Read the model definition and answer for the solid it produces. Units are mm, in the model's axes. A direction names the side the tool comes from. Round coordinates to 2 decimals unless told otherwise and drop trailing zeros. Order: outer loops, then holes, each group sorted by start corner. A loop starts at its lowest first (then second) coordinate and runs counter-clockwise, first axis right, second up. Notation, with made-up numbers: (24.5, -29) -> (41.5, -29) arc R31 ccw to (41.5, 1) -> close; hole circle Ø10 at (50.5, 46.5). An arc over 180 degrees is marked (long way). Answer as a JSON object with one key per item and string values. Group by question number.
Item 1: The mould has two halves that part along Z. Classify faces 1 (the flat face through (16, -8, 48)), 2 (the flat face through (16, -8, 32)), 3 (the flat face through (32, -8, 24)), 4 (the flat face through (16, -8, 0)): pulls with the +Z half, pulls with the -Z half, needs draft (parallel to the pull), parting line crosses it, or undercut.
Item 2: Given P1, Ø4, axis at x = 20.5, z = 41.5, coming from the -Y side, flat-ended and moving along its own axis, determine where the tip first touches the part or whether it passes through.
Item 3: Section B-B, the plane z = 16 is taken. Write down the section's boundary in (x, y), plus the area to 3 significant figures.
Item 4: Section C-C, the plane x = 25 is taken. Write down the section's boundary in (y, z).
Item 5: Consider probe 1 along Z at (x, y) = (4.5, -11.5); probe 2 along X at (y, z) = (-11, 23.5); probe 3 along Y at (x, z) = (9, 39.5). Determine where each line is inside the solid, lowest interval first. Write a range as from..to.
Item 6: For faces 5 (the flat face through (0, -8, 24)), 6 (the flat face through (1, -8, 25)), determine the directions among +Z, -Z, +X, -X, +Y, -Y from which every point of the face is accessible in a straight line to the end or side of a thin tool.
Item 7: Section A-A, the plane y = -10.25 is taken. Write down the section's boundary in (x, z).
from build123d import *

# Parameters (mm, degrees)
F0_W     = 32
F0_H     = 48
F0_W_2   = 30
F0_H_2   = 15
F0_H_3   = 14
F1_DEPTH = 17
F2_W     = 32
F2_H     = 48
F3_DEPTH = 1


with BuildPart() as f1:
    # F0 (on Front) → F1 (new body)
    with BuildSketch(Plane.XZ):
        with Locations((16, 24)):
            Rectangle(F0_W, F0_H)
        with Locations((16, 9.5)):
            Rectangle(F0_W_2, F0_H_2, mode=Mode.SUBTRACT)
        with Locations((16, 25)):
            Rectangle(F0_W_2, F0_H_3, mode=Mode.SUBTRACT)
        with Locations((16, 40)):
            Rectangle(F0_W_2, F0_H_3, mode=Mode.SUBTRACT)
    extrude(amount=F1_DEPTH)

    # F2 (on Front) → F3 (join)
    with BuildSketch(Plane.XZ):
        with Locations((16, 24)):
            Rectangle(F2_W, F2_H)
    extrude(amount=-F3_DEPTH)


solid = f1.part
Values found:
{
 "1": {"face 1": "pulls with the +Z half", "face 2": "undercut", "face 3": "needs draft", "face 4": "pulls with the -Z half"},
 "2": {"P1": "y = 0"},
 "3": {"outline": "(0, -17) -> (1, -17) -> (1, 0) -> (31, 0) -> (31, -17) -> (32, -17) -> (32, 1) -> (0, 1) -> close", "area": "66.0 mm2"},
 "4": {"outline": "(-17, 0) -> (1, 0) -> (1, 48) -> (-17, 48) -> (-17, 47) -> (0, 47) -> (0, 33) -> (-17, 33) -> (-17, 32) -> (0, 32) -> (0, 18) -> (-17, 18) -> (-17, 17) -> (0, 17) -> (0, 2) -> (-17, 2) -> close"},
 "5": {"probe 1": "0..2, 17..18, 32..33, 47..48", "probe 2": "0..1, 31..32", "probe 3": "0..1"},
 "6": {"face 5": "+Z, -Z, -X, +Y, -Y", "face 6": "-Y"},
 "7": {"outline": "(0, 0) -> (32, 0) -> (32, 48) -> (0, 48) -> close; hole (1, 2) -> (31, 2) -> (31, 17) -> (1, 17) -> close; hole (1, 18) -> (31, 18) -> (31, 32) -> (1, 32) -> close; hole (1, 33) -> (31, 33) -> (31, 47) -> (1, 47) -> close"}
}
